from build123d import *

# Parameters (mm, degrees)
SKETCH_1_R          = 12.9
EXTRUDE_1_DEPTH     = 8.3
SKETCH_2_R          = 6
EXTRUDE_2_DEPTH     = 4.5
SKETCH_3_R          = 4.025
CUT_EXTRUDE_1_DEPTH = 25
EXTRUDE_3_DEPTH     = 4
SKETCH_6_R          = 2.55
CUT_EXTRUDE_3_DEPTH = 13.8
SKETCH_7_R          = 4.025
CUT_EXTRUDE_4_DEPTH = 13.8


with BuildPart() as part:
    # 草图1 → 凸台-拉伸1 (new body)
    with BuildSketch(Plane.XY):
        Circle(SKETCH_1_R)
    extrude(amount=EXTRUDE_1_DEPTH)

    # 草图2 → 凸台-拉伸2 (add)
    with BuildSketch(Plane.XY.offset(8.3)):
        Circle(SKETCH_2_R)
    extrude(amount=EXTRUDE_2_DEPTH)

    # 草图3 → 切除-拉伸1 (cut)
    with BuildSketch(Plane.XY.offset(12.8)):
        Circle(SKETCH_3_R)
    extrude(amount=-CUT_EXTRUDE_1_DEPTH, mode=Mode.SUBTRACT)

    # 草图4 → 凸台-拉伸3 (add)
    with BuildSketch(Plane(origin=(0, 0, 0), x_dir=(-1, 0, 0), z_dir=(0, 0, -1))):
        with BuildLine():
            Line((-5.057343549, 11.867319673), (-20.2907969, 5.375474071))
            ThreePointArc((-20.2907969, 5.375474071), (-23.843241559, 0), (-20.2907969, -5.375474071))
            Line((-20.2907969, -5.375474071), (-5.057343549, -11.867319673))
            ThreePointArc((-5.057343549, -11.867319673), (0, -12.9), (5.057343549, -11.867319673))
            Line((5.057343549, -11.867319673), (20.2907969, -5.375474071))
            ThreePointArc((20.2907969, -5.375474071), (23.843241559, 0), (20.2907969, 5.375474071))
            Line((20.2907969, 5.375474071), (5.057343549, 11.867319673))
            ThreePointArc((5.057343549, 11.867319673), (0, 12.9), (-5.057343549, 11.867319673))
        make_face()
    extrude(amount=-EXTRUDE_3_DEPTH)

    # 草图6 → 切除-拉伸3 (cut, through all)
    with BuildSketch(Plane(origin=(0, 0, 0), x_dir=(-1, 0, 0), z_dir=(0, 0, -1))):
        with Locations((-18, 0)):
            Circle(SKETCH_6_R)
        with Locations((18, 0)):
            Circle(SKETCH_6_R)
    extrude(amount=-CUT_EXTRUDE_3_DEPTH, mode=Mode.SUBTRACT)

    # 草图7 → 切除-拉伸4 (cut, through all)
    with BuildSketch(Plane(origin=(0, 0, 0), x_dir=(-1, 0, 0), z_dir=(0, 0, -1))):
        Circle(SKETCH_7_R)
    extrude(amount=-CUT_EXTRUDE_4_DEPTH, mode=Mode.SUBTRACT)


solid = part.part
Geometry check sheet. Reference: the model listing, model coordinates, mm. A direction names the side the tool comes from. Round coordinates to 2 decimals unless told otherwise and drop trailing zeros. Loops run counter-clockwise (first coordinate to the right, second up) from the corner with the lowest first, then second, coordinate; pieces in that order, holes last.
Item 1: Mould release check, pull along Y, two halves, no side actions. Record for faces 3 (the cylindrical face through (-15.452, 0.112, 1.972)), 4 (the flat face through (12.567, 8.667, 1.972)), 5 (the cylindrical face through (20.548, 0.112, 1.972)), 6 (the flat face through (12.781, -8.576, 1.972)): pulls with the +Y half, pulls with the -Y half, needs draft (parallel to the pull), parting line crosses it, or undercut.
Item 2: Access from +Z, -Z, +X, -X, +Y, -Y to the whole of each face (thin tool, end or side, straight path). Record for faces 1 (the flat face through (6, -3, 8.3)), 2 (the flat face through (-12.781, 8.576, 1.972)).
Item 3: Thickness scan on line 1 (Y direction, x = 0, z = 2.3) (3 decimals); line 2 (Z direction, x = 13.5, y = -6.75); line 3 (Y direction, x = -18, z = 1.8). Record the ranges inside material, lowest first.
Item 4: Gauge pin test, flat ends, axial feed: pin 1 (9.5 mm diameter, centred on x = 11.5, y = 0, fed in from +Z); pin 2 (3 mm diameter, centred on x = -19, y = -0.5, fed in from +Z); pin 3 (2 mm diameter, centred on x = 6, z = 4.5, fed in from -Y). Record the tip position at first contact, or that the pin passes through.
Item 5: Cross-section at D-D on z = 5. Record the boundary of the cut face in (x, y) (3 decimals), then the cut area to 3 significant figures.
Item 6: Cross-section at A-A on x = 0. Record the boundary of the cut face in (y, z) (3 decimals), then the cut area to 3 significant figures.
Item 7: Cross-section at C-C on z = 1.25. Record the boundary of the cut face in (x, y) (3 decimals), then the cut area to 3 significant figures.
Item 8: Cross-section at B-B on y = 1. Record the boundary of the cut face in (x, z), then the cut area to 3 significant figures.
Answer sheet:
1. face 3: undercut
1. face 4: pulls with the +Y half
1. face 5: undercut
1. face 6: pulls with the -Y half
2. face 1: +Z
2. face 2: +Z, -Z, -X, +Y
3. line 1: y = -12.9 to -4.025, 4.025 to 12.9
3. line 2: z = 0 to 4
3. line 3: y = -6.35 to -2.55, 2.55 to 6.35
4. pin 1: stops at z = 8.3
4. pin 2: stops at z = 4
4. pin 3: stops at y = -11.89
5. outline: circle Ø25.8 at (0, 0); hole circle Ø8.05 at (0, 0)
5. area: 472 mm2
6. outline: (-12.9, 0) - (-4.025, 0) - (-4.025, 12.8) - (-6, 12.8) - (-6, 8.3) - (-12.9, 8.3) - close; (4.025, 0) - (12.9, 0) - (12.9, 8.3) - (6, 8.3) - (6, 12.8) - (4.025, 12.8) - close
6. area: 165 mm2
7. outline: (-20.291, -5.375) - (-5.057, -11.867) arc R12.9 ccw to (5.057, -11.867) - (20.291, -5.375) arc R5.843 ccw to (20.291, 5.375) - (5.057, 11.867) arc R12.9 ccw to (-5.057, 11.867) - (-20.291, 5.375) arc R5.843 ccw to start; hole circle Ø5.1 at (-18, 0); hole circle Ø8.05 at (0, 0); hole circle Ø5.1 at (18, 0)
7. area: 743 mm2
8. outline: (-23.76, 0) - (-20.35, 0) - (-20.35, 4) - (-23.76, 4) - close; (-15.65, 0) - (-3.9, 0) - (-3.9, 12.8) - (-5.92, 12.8) - (-5.92, 8.3) - (-12.86, 8.3) - (-12.86, 4) - (-15.65, 4) - close; (3.9, 0) - (15.65, 0) - (15.65, 4) - (12.86, 4) - (12.86, 8.3) - (5.92, 8.3) - (5.92, 12.8) - (3.9, 12.8) - close; (20.35, 0) - (23.76, 0) - (23.76, 4) - (20.35, 4) - close
8. area: 217 mm2
